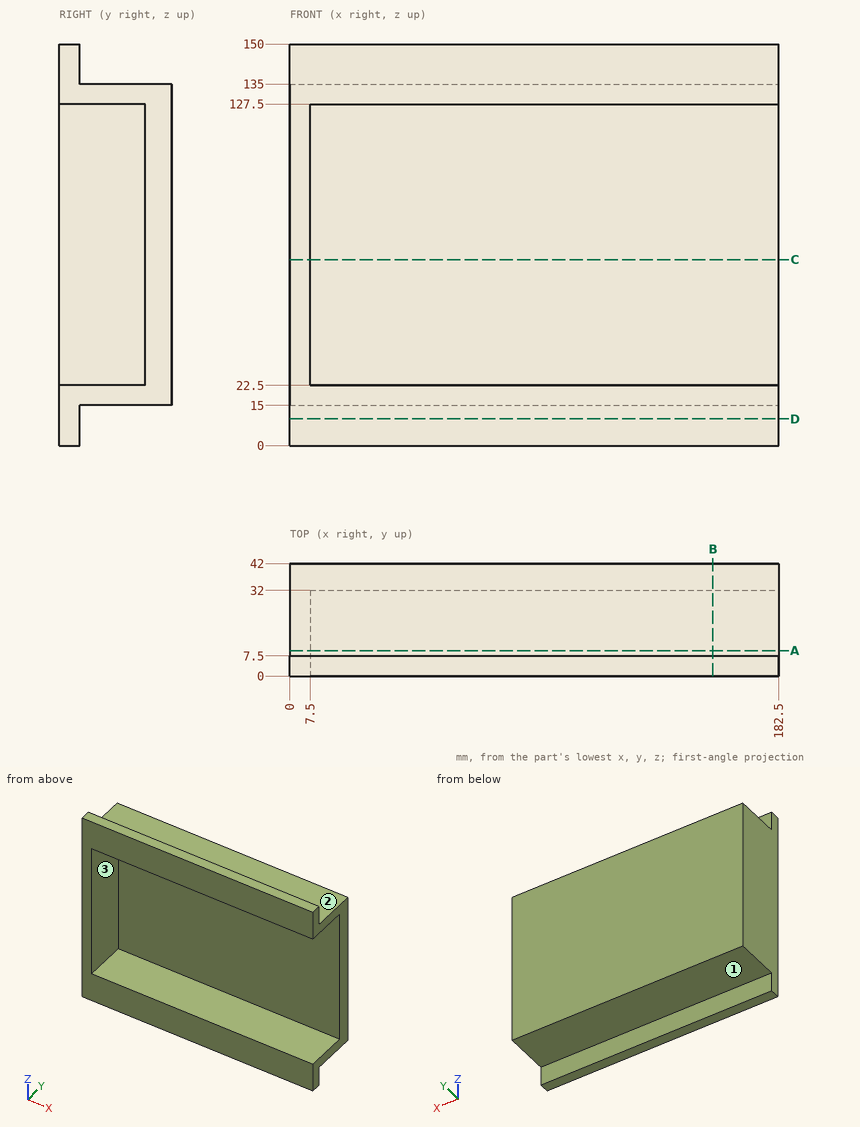
Part print with two shaded views. Sizes in mm from the minimum x, y, z corner. A direction names the side the tool comes from. Round coordinates to 2 decimals unless told otherwise and drop trailing zeros. Order: outer loops, then holes, each group sorted by start corner. A loop starts at its lowest first (then second) coordinate and runs counter-clockwise, first axis right, second up. Notation, with made-up numbers: M 58,-1.75 L 85,-1.75 A9 ccw 85,7.25 Z; hole C 13.5,32.25 d11. An arc over 180 degrees is marked long. Use CSV: the item, a comma, the result in double quotes. Start each with the question number.
(1) Cut at B-B on x = 158. List the corners of the cut face in (y, z).
(2) Cut at A-A on y = 9.5. List the corners of the cut face in (x, z).
(3) Cut at D-D on z = 10. List the corners of the cut face in (x, y), then the cut area to 3 significant figures.
(4) Cut at C-C on z = 69.5. List the corners of the cut face in (x, y), then the cut area to 4 significant figures.
(5) Drill centre lines: probe 1 along Z at (x, y) = (75.5, 4); probe 2 along Z at (x, y) = (93, 13); probe 3 along Y at (x, z) = (52, 100). Where is each one in solid material? Low to high.
(6) Flat gauge pins, fed straight in: P1, Ø16.5, axis at x = 81.5, z = 8.5, coming from the +Y side; P2, Ø17, axis at x = 122, y = 18.5, coming from the +Z side; P3, Ø17, axis at x = 84.5, y = 25, coming from the -Z side; P4, Ø2, axis at y = 14, z = 65, coming from the +X side. Where does each tip first touch, or does it go through?
(7) Tool access for the marked faces 1, 2 and 3: list every direction of +Z, -Z, +X, -X, +Y, -Y with a clear straight run to the whole face (end or side of a thin tool).
Findings:
1,outline,"M 0,0 L 7.5,0 L 7.5,15 L 42,15 L 42,135 L 7.5,135 L 7.5,150 L 0,150 L 0,127.5 L 32,127.5 L 32,22.5 L 0,22.5 Z"
2,outline,"M 0,15 L 182.5,15 L 182.5,22.5 L 7.5,22.5 L 7.5,127.5 L 182.5,127.5 L 182.5,135 L 0,135 Z"
3,outline,"M 0,0 L 182.5,0 L 182.5,7.5 L 0,7.5 Z"
3,area,"1,370 mm^2"
4,outline,"M 0,0 L 7.5,0 L 7.5,32 L 182.5,32 L 182.5,42 L 0,42 Z"
4,area,"2,065 mm^2"
5,probe 1,"z = 0 to 22.5, 127.5 to 150"
5,probe 2,"z = 15 to 22.5, 127.5 to 135"
5,probe 3,"y = 32 to 42"
6,P1,"stops at y = 42"
6,P2,"stops at z = 135"
6,P3,"stops at z = 15"
6,P4,"stops at x = 7.5"
7,face 1,"-Z, +X, -X, +Y"
7,face 2,"+Z, +X, -X, +Y"
7,face 3,"+X, -Y"
